```python
from build123d import *

# Parameters (mm, degrees)
BOSS_EXTRUDE1_DEPTH = 115
CUT_EXTRUDE1_DEPTH  = 115
CUT_EXTRUDE2_START  = 7.5
CUT_EXTRUDE2_DEPTH  = 100
CUT_EXTRUDE3_START  = 7.5
CUT_EXTRUDE3_DEPTH  = 100
CUT_EXTRUDE4_REACH  = 260.68
SKETCH6_W           = 70.076051312
SKETCH6_H           = 19.92290321
CUT_EXTRUDE5_REACH  = 293.015
SKETCH5_W           = 70
SKETCH5_H           = 20.313376992
CUT_EXTRUDE6_REACH  = 334.213
SKETCH7_W           = 70
SKETCH7_H           = 17.498886338
FILLET1_R           = 15


# Read off the part's stored shape, not the designer's step: Cut-Extrude2, Cut-Extrude3
with BuildPart() as part:
    # Sketch1 → Boss-Extrude1 (new body)
    with BuildSketch(Plane(origin=(0, 0, 0), x_dir=(0, 0, -1), z_dir=(1, 0, 0))):
        with BuildLine():
            Line((89.8548345, 121.890508387), (339.8548345, 121.890508387))
            Line((339.8548345, 121.890508387), (339.8548345, 142.698803067))
            Line((339.8548345, 142.698803067), (328.974757131, 148.244473571))
            Line((328.974757131, 148.244473571), (304.07146893, 160.937897169))
            Line((304.07146893, 160.937897169), (291.499350701, 165.900575417))
            ThreePointArc((291.499350701, 165.900575417), (280.939522904, 169.403551358), (270.055923817, 171.711813574))
            Line((270.055923817, 171.711813574), (268.171463935, 172.003048284))
            ThreePointArc((268.171463935, 172.003048284), (254.466056361, 173.586145336), (240.679656072, 174.114879761))
            Line((240.679656072, 174.114879761), (232.021178794, 174.114879761))
            Line((232.021178794, 174.114879761), (204.700095622, 174.114879761))
            Line((204.700095622, 174.114879761), (181.005704906, 172.180643784))
            Line((181.005704906, 172.180643784), (169.793278807, 169.525069181))
            ThreePointArc((169.793278807, 169.525069181), (162.738148163, 167.508293641), (155.897481651, 164.85357451))
            Line((155.897481651, 164.85357451), (139.701268702, 157.697108323))
            ThreePointArc((139.701268702, 157.697108323), (131.522677332, 153.88092637), (123.507487012, 149.732513946))
            Line((123.507487012, 149.732513946), (122.849499947, 149.374661332))
            ThreePointArc((122.849499947, 149.374661332), (105.217865801, 137.440006065), (90.215677989, 122.332230589))
            Line((90.215677989, 122.332230589), (89.8548345, 121.890508387))
        make_face()
    extrude(amount=BOSS_EXTRUDE1_DEPTH)

    # Sketch2 → Cut-Extrude1 (cut)
    with BuildSketch(Plane(origin=(115, 0, 0), x_dir=(0, 0, -1), z_dir=(1, 0, 0))):
        with BuildLine():
            Line((113.475739659, 133.359325966), (201.174236889, 137.018348058))
            Line((201.174236889, 137.018348058), (207.075885424, 168.415118264))
            Line((207.075885424, 168.415118264), (192.666474105, 167.813918061))
            Line((192.666474105, 167.813918061), (190.829871081, 167.73728994))
            ThreePointArc((190.829871081, 167.73728994), (182.233808887, 166.844681368), (173.813252446, 164.899619793))
            Line((173.813252446, 164.899619793), (169.2892062, 163.555605085))
            ThreePointArc((169.2892062, 163.555605085), (160.569837528, 160.5967142), (152.103009161, 156.977979241))
            Line((152.103009161, 156.977979241), (131.888883088, 147.40524948))
            Line((131.888883088, 147.40524948), (120.054289503, 140.950016615))
            ThreePointArc((120.054289503, 140.950016615), (116.601738736, 138.565427019), (113.722697716, 135.512969462))
            Line((113.722697716, 135.512969462), (113.475739659, 135.188837012))
            Line((113.475739659, 135.188837012), (113.475739659, 133.359325966))
        make_face()
        with BuildLine():
            Line((221.003775967, 168.415118264), (218.761149524, 138.906875589))
            Line((218.761149524, 138.906875589), (272.584184163, 138.906875589))
            Line((272.584184163, 138.906875589), (274.383679522, 162.58444611))
            Line((274.383679522, 162.58444611), (267.028526617, 163.966993649))
            Line((267.028526617, 163.966993649), (257.016670223, 165.848921543))
            Line((257.016670223, 165.848921543), (255.744876296, 166.087980551))
            ThreePointArc((255.744876296, 166.087980551), (245.628472921, 167.506912168), (235.424062848, 167.981253005))
            Line((235.424062848, 167.981253005), (234.695600568, 167.981253005))
            Line((234.695600568, 167.981253005), (221.003775967, 168.415118264))
        make_face()
        with BuildLine():
            Line((276.275786009, 160.987395212), (275.646964577, 141.143186512))
            Line((275.646964577, 141.143186512), (283.14790924, 141.143186512))
            Line((283.14790924, 141.143186512), (294.416525801, 147.803376186))
            Line((294.416525801, 147.803376186), (296.046101937, 148.766518919))
            ThreePointArc((296.046101937, 148.766518919), (296.405855365, 149.13182216), (296.537289859, 149.627396535))
            Line((296.537289859, 149.627396535), (296.537289859, 150.540124257))
            ThreePointArc((296.537289859, 150.540124257), (296.433404588, 150.983946735), (296.143333074, 151.335555977))
            Line((296.143333074, 151.335555977), (294.416525801, 152.651218661))
            Line((294.416525801, 152.651218661), (277.097452917, 160.987395212))
            Line((277.097452917, 160.987395212), (276.275786009, 160.987395212))
        make_face()
    extrude(amount=-CUT_EXTRUDE1_DEPTH, mode=Mode.SUBTRACT)

    # Cut-Extrude2 outline → Cut-Extrude2 (cut)
    with BuildSketch(Plane.YZ.offset(CUT_EXTRUDE2_START)):
        with BuildLine():
            Line((121.890508387, -99.688159251), (121.890508387, -171.289102204))
            Line((121.890508387, -171.289102204), (135.747336393, -170.710957294))
            Line((135.747336393, -170.710957294), (133.359325966, -113.475739659))
            Line((133.359325966, -113.475739659), (135.188837012, -113.475739659))
            Line((135.188837012, -113.475739659), (135.512969462, -113.722697716))
            ThreePointArc((135.512969462, -113.722697716), (138.565427019, -116.601738736), (140.950016615, -120.054289503))
            Line((140.950016615, -120.054289503), (147.40524948, -131.888883088))
            Line((147.40524948, -131.888883088), (156.977979241, -152.103009161))
            ThreePointArc((156.977979241, -152.103009161), (160.5967142, -160.569837528), (163.555605085, -169.2892062))
            Line((163.555605085, -169.2892062), (163.632345036, -169.547518172))
            Line((163.632345036, -169.547518172), (169.408178174, -169.306534555))
            ThreePointArc((169.408178174, -169.306534555), (167.428165725, -162.501028912), (164.85357451, -155.897481651))
            Line((164.85357451, -155.897481651), (157.697108323, -139.701268702))
            ThreePointArc((157.697108323, -139.701268702), (153.88092637, -131.522677332), (149.732513946, -123.507487012))
            Line((149.732513946, -123.507487012), (149.374661332, -122.849499947))
            ThreePointArc((149.374661332, -122.849499947), (141.537958861, -110.480020928), (132.127738515, -99.261033903))
            Line((132.127738515, -99.261033903), (121.890508387, -99.688159251))
        make_face()
    extrude(amount=CUT_EXTRUDE2_DEPTH, mode=Mode.SUBTRACT)

    # Cut-Extrude3 outline → Cut-Extrude3 (cut)
    with BuildSketch(Plane.YZ.offset(CUT_EXTRUDE3_START)):
        with BuildLine():
            Line((121.890508387, -291.499350701), (121.890508387, -333.35633566))
            Line((121.890508387, -333.35633566), (146.011144709, -333.35633566))
            Line((146.011144709, -333.35633566), (160.937897169, -304.07146893))
            Line((160.937897169, -304.07146893), (165.900575417, -291.499350701))
            Line((165.900575417, -291.499350701), (154.055340396, -291.499350701))
            Line((154.055340396, -291.499350701), (152.651218661, -294.416525801))
            Line((152.651218661, -294.416525801), (151.335555977, -296.143333074))
            ThreePointArc((151.335555977, -296.143333074), (150.983946735, -296.433404588), (150.540124257, -296.537289859))
            Line((150.540124257, -296.537289859), (149.627396535, -296.537289859))
            ThreePointArc((149.627396535, -296.537289859), (149.13182216, -296.405855365), (148.766518919, -296.046101937))
            Line((148.766518919, -296.046101937), (146.079212499, -291.499350701))
            Line((146.079212499, -291.499350701), (121.890508387, -291.499350701))
        make_face()
    extrude(amount=CUT_EXTRUDE3_DEPTH, mode=Mode.SUBTRACT)

    # Cut-Extrude4: up to this plane
    cut_extrude4_end = Plane(origin=(0, 137.018348058, -201.174236889), z_dir=(0, -0.18473466771426061, -0.9827884322398701))
    # Sketch6 → Cut-Extrude4 (cut, up to the surface)
    with BuildSketch(Plane(origin=(0, -15.732649467, -207.008545619), x_dir=(-1, 0, 0), z_dir=(0, -0.07578145826840303, -0.9971244509000441)), mode=Mode.PRIVATE) as cut_extrude4_sk1:
        with Locations((-57.714978641, 162.925898332)):
            Rectangle(SKETCH6_W, SKETCH6_H)
    cut_extrude4_tool1 = split(extrude(cut_extrude4_sk1.sketch, amount=-CUT_EXTRUDE4_REACH, mode=Mode.PRIVATE), bisect_by=cut_extrude4_end, keep=Keep.BOTH, mode=Mode.PRIVATE)
    add(cut_extrude4_tool1.solids().sort_by_distance((57.714979, 146.724747, -219.355308))[0], mode=Mode.SUBTRACT)

    # Cut-Extrude5: up to this plane
    cut_extrude5_end = Plane(origin=(0, 168.415118264, -221.003775967), z_dir=(0, 0.07578145826840302, 0.9971244509000441))
    # Sketch5 → Cut-Extrude5 (cut, up to the surface)
    with BuildSketch(Plane(origin=(0, -31.848196468, -169.432405211), x_dir=(1, 0, 0), z_dir=(0, 0.18473466771426064, 0.9827884322398701)), mode=Mode.PRIVATE) as cut_extrude5_sk1:
        with Locations((57.5, 181.980591777)):
            Rectangle(SKETCH5_W, SKETCH5_H)
    cut_extrude5_tool1 = split(extrude(cut_extrude5_sk1.sketch, amount=-CUT_EXTRUDE5_REACH, mode=Mode.PRIVATE), bisect_by=cut_extrude5_end, keep=Keep.BOTH, mode=Mode.PRIVATE)
    add(cut_extrude5_tool1.solids().sort_by_distance((57.5, 147.000224, -203.050529))[0], mode=Mode.SUBTRACT)

    # Cut-Extrude6: up to this plane
    cut_extrude6_end = Plane(origin=(115, 121.890508387, -89.8548345), z_dir=(0, 1, 0))
    # Sketch7 → Cut-Extrude6 (cut, up to the surface)
    with BuildSketch(Plane(origin=(0, 168.866544526, -31.741831678), x_dir=(1, 0, 0), z_dir=(0, 0.9827884322398701, -0.18473466771426067)), mode=Mode.PRIVATE) as cut_extrude6_sk1:
        with Locations((57.5, 181.149117049)):
            Rectangle(SKETCH7_W, SKETCH7_H)
    cut_extrude6_tool1 = split(extrude(cut_extrude6_sk1.sketch, amount=-CUT_EXTRUDE6_REACH, mode=Mode.PRIVATE), bisect_by=cut_extrude6_end, keep=Keep.BOTH, mode=Mode.PRIVATE)
    add(cut_extrude6_tool1.solids().sort_by_distance((57.5, 135.402023, -209.773088))[0], mode=Mode.SUBTRACT)

    # Fillet1
    fillet1_edges = [part.edges().sort_by_distance(p)[0] for p in [
        (115, 132.294655727, -339.8548345),
        (0, 132.294655727, -339.8548345),
    ]]
    fillet(fillet1_edges, radius=FILLET1_R)


solid = part.part
```
CAD build for the part. Positions are in the model's coordinates, mm. A direction names the side the tool comes from. Coordinates: 2 decimals unless noted, no trailing zeros. Order: outer loops, then holes, each group sorted by start corner. A loop starts at its lowest first (then second) coordinate and runs counter-clockwise, first axis right, second up. Notation, with made-up numbers: (-25, -37.75) -> (-14, -37.75) arc R20 ccw to (-14, -8.75) -> close; hole circle Ø11 at (64, 15). An arc over 180 degrees is marked (long way). Use one line per item in the form item = value. Start each with the question number.
1) Tool access for faces 1 (the flat face through (57, 121.891, -241)), 2 (the cylindrical face through (58.305, 166.864, -182.353)), 3 (the flat face through (57.01, 129.56, -199.772)), 4 (the flat face through (115, 137, -232)), 5 (the flat face through (57, 134, -333.356)): list every direction of +Z, -Z, +X, -X, +Y, -Y with a clear straight run to the whole face (end or side of a thin tool).
2) Pull direction Y, two halves, no side cores. Call faces 6 (the flat face through (107.5, 129, -135)), 7 (the flat face through (56.8, 166.48, -169.43)), 8 (the flat face through (58.21, 157.22, -212.7)): +Y half, -Y half, draft (parallel to the pull), parting line (faces both ways), or undercut.
3) Band-saw the part on B-B on x = 84.5. State how many separate pieces and enclosed holes the cut face has, then the cut area to 3 significant figures.
4) Band-saw the part on C-C on z = -129.5. Give the cut face in (x, y).
5) Band-saw the part on A-A on z = -316. Give the cut face in (x, y), then the cut area to 3 significant figures.
6) Drill centre lines: L1, parallel to Z at x = 26, y = 159; L2, parallel to X at y = 132, z = -218; L3, parallel to X at y = 138.5, z = -215.5. Where is each one in solid material? Low to high. Write a range as [from, to].
7) Drop flat-ended pins along their axis: pin 1 (19.5 mm diameter, centred on x = 52.5, y = 135.5, fed in from +Z); pin 2 (1.5 mm diameter, centred on x = 110.5, y = 134, fed in from -Z); pin 3 (8.5 mm diameter, centred on x = 82.5, z = -281, fed in from +Y); pin 4 (10 mm diameter, centred on y = 168, z = -299, fed in from -X). Give the stop position or say it passes through.
Entries:
q1.face_1 = +Z, -Z, +X, -X, -Y
q1.face_2 = +X, -X
q1.face_3 = -Y
q1.face_4 = +Z, -Z, +X, +Y, -Y
q1.face_5 = +Y, -Y
q2.face_6 = draft
q2.face_7 = -Y half
q2.face_8 = undercut
q3.separate_pieces = 4
q3.enclosed_holes = 0
q3.area = 2,980 mm2
q4.outline = (0, 121.89) -> (7.5, 121.89) -> (7.5, 134.03) -> (0, 134.03) -> close; (0, 146.1) -> (7.5, 146.1) -> (7.5, 152.87) -> (0, 152.87) -> close; (107.5, 121.89) -> (115, 121.89) -> (115, 134.03) -> (107.5, 134.03) -> close; (107.5, 146.1) -> (115, 146.1) -> (115, 152.87) -> (107.5, 152.87) -> close
q5.outline = (0, 121.89) -> (7.5, 121.89) -> (7.5, 154.86) -> (0, 154.86) -> close; (107.5, 121.89) -> (115, 121.89) -> (115, 154.86) -> (107.5, 154.86) -> close
q5.area = 495 mm2
q6.L1 = [-291.5, -281.23], [-276.21, -274.11], [-220.29, -205.31]
q6.L2 = [0, 22.5], [92.5, 115]
q6.L3 = [0, 22.5], [92.75, 115]
q7.pin_1 = -93.13
q7.pin_2 = -336.25
q7.pin_3 = 170.44
q7.pin_4 = 0
